Read the model definition and answer for the solid it produces. Units are mm, in the model's axes. A direction names the side the tool comes from. Give positions to 0.01 mm unless a question says otherwise; leave off trailing zeros. Write each loop counter-clockwise with the first axis right and the second up, starting at its lowest first coordinate (ties: lowest second). Pieces come first, ordered by that corner, then holes. Notation, with made-up numbers: M -34.5,-38.75 L -21.5,-38.75 A10 cw -21.5,-28.75 Z; hole C 82.5,-10.5 d8. An arc over 180 degrees is marked long. Use a Markdown table: item, result. Add a question column.
Item 1: Given P1, Ø2, axis at x = 1.5, z = -27.5, coming from the -Y side; P2, Ø2, axis at x = -5.5, z = -20, coming from the -Y side; P3, Ø1, axis at x = 2.5, z = -18, coming from the +Y side, each flat-ended and moving along its own axis, determine where each tip first touches the part or whether it passes through.
Item 2: A cutting plane is placed at A-A on x = 0. Determine the outline of the cut face in (y, z).
Item 3: Consider probe 1 along Z at (x, y) = (0, -2); probe 2 along X at (y, z) = (-3, -26); probe 3 along Z at (x, y) = (5.75, 7.5). Determine where each line is inside the solid, lowest interval first. Write a range as [from, to].
Item 4: A cutting plane is placed at B-B on y = 0. Determine the outline of the cut face in (x, z).
Item 5: For faces 4 (the flat face through (0, 0, -32)), 5 (the cylindrical face through (5.723, 1.802, -15.776)), determine the directions among +Z, -Z, +X, -X, +Y, -Y from which every point of the face is accessible in a straight line to the end or side of a thin tool.
Item 6: A cutting plane is placed at D-D on x = -8. Determine the outline of the cut face in (y, z), then the cut area to 3 significant figures.
Item 7: A cutting plane is placed at C-C on z = -8. Determine the outline of the cut face in (x, y), then the cut area to 3 significant figures.
Item 8: The mould has two halves that part along Z. Classify faces 1 (the flat face through (7, 0, 0)), 2 (the cylindrical face through (-0.195, -0.084, -24.513)), 3 (the cylindrical face through (-2.17, 9.76, 1.97)): pulls with the +Z half, pulls with the -Z half, needs draft (parallel to the pull), parting line crosses it, or undercut.
Solid Edge part; units mm, degrees
sketch "Sketch1" plane through (0, 0, 0) normal (0, 0, 1) x (1, 0, 0)
  circle A0 centre (0, 0) radius 10
extrude "Protrusion1" add sketch "Sketch1" along normal blind 4
sketch "Sketch2" plane through (0, 0, 0) normal (0, 0, 1) x (1, 0, 0)
  circle A0 centre (0, 0) radius 6
extrude "ExtrudedProtrusion_2" add sketch "Sketch2" against normal blind 32
sketch "Sketch3" plane through (0, 0, 0) normal (0, -1, 0) x (1, 0, 0)
  circle A0 centre (0, -26) radius 1.5
extrude "ExtrudedCutout_1" cut sketch "Sketch3" along normal mid plane 639.6165
properties part number "8"
Filled in:
| question | item | result |
|---|---|---|
| 1 | P1 | y = -5.98 |
| 1 | P2 | y = -3.97 |
| 1 | P3 | y = 5.66 |
| 2 | outline | M -10,0 L -6,0 L -6,-24.5 L 6,-24.5 L 6,0 L 10,0 L 10,4 L -10,4 Z; M -6,-32 L 6,-32 L 6,-27.5 L -6,-27.5 Z |
| 3 | probe 1 | [-32, -27.5], [-24.5, 4] |
| 3 | probe 2 | [-5.2, -1.5], [1.5, 5.2] |
| 3 | probe 3 | [0, 4] |
| 4 | outline | M -10,0 L -6,0 L -6,-32 L 6,-32 L 6,0 L 10,0 L 10,4 L -10,4 Z; hole C 0,-26 d3 |
| 5 | face 4 | -Z, +X, -X, +Y, -Y |
| 5 | face 5 | -Z |
| 6 | outline | M -6,0 L 6,0 L 6,4 L -6,4 Z |
| 6 | area | 48.0 mm² |
| 7 | outline | C 0,0 d12 |
| 7 | area | 113 mm² |
| 8 | face 1 | pulls with the -Z half |
| 8 | face 2 | undercut |
| 8 | face 3 | needs draft |
